Work out the finished part from the listing and answer in its coordinate system (mm). A direction names the side the tool comes from. Give positions to 0.01 mm unless a question says otherwise; leave off trailing zeros. Order: outer loops, then holes, each group sorted by start corner. A loop starts at its lowest first (then second) coordinate and runs counter-clockwise, first axis right, second up. Notation, with made-up numbers: (0.25, -0.5) - (42.25, -0.5) arc R21 ccw to (42.25, 31.5) - close; hole circle Ø5 at (-33, 42). An arc over 180 degrees is marked (long way). Write each question's results on one line, items separated by ' | '.
from build123d import *

# Parameters (mm, degrees)
F3_R = 12.7
F4_T = -2.54


with BuildPart() as f2:
    # F0 (on Front) → F2 (revolve)
    with BuildSketch(Plane.XZ):
        Polygon((0, -76.0418921709), (0, 76.0156810284), (-8.6687002331, 76.3955637813), (-8.6687002331, 59.0391717851), (-31.3122980297, 40.9342460334), (-31.3122980297, -76.0418921709), align=None)
    revolve(axis=Axis((1.9537888002, 0, -0.1578219235), (0, 0, -1)))

    # F3
    f3_edges = [f2.edges().sort_by_distance(p)[0] for p in [
        (35.219876, 0, 40.934246),
        (12.576278, 0, 59.039172),
    ]]
    fillet(f3_edges, radius=F3_R)

    # F4
    f4_openings = [f2.faces().sort_by_distance(p)[0] for p in [
        (8.241928, 0, 76.205622),
    ]]
    offset(amount=F4_T, openings=f4_openings)


solid = f2.part
1. A cutting plane is placed at B-B, the plane z = 31. Write down the section's boundary in (x, y), then the cut area to 3 significant figures.
Answer list:
outline: circle Ø66.53 at (1.95, 0); circle Ø8.99 at (1.95, 0); hole circle Ø61.45 at (1.95, 0); hole circle Ø3.91 at (1.95, 0) | area: 562 mm^2
2. Given P1, Ø3, axis at x = -6, z = -29, coming from the -Y side; P2, Ø4, axis at y = 22, z = 18, coming from the +X side; P3, Ø1, axis at x = -20.5, z = 21.5, coming from the +Y side, each flat-ended and moving along its own axis, determine where each tip first touches the part or whether it passes through.
Answer list:
P1: y = -32.63 | P2: x = 28.54 | P3: y = 24.99
3. Determine the mould class of faces 4 (the face through (-29.776, 9.992, -21.383)), 5 (the face through (2, -7, -76.042)), 6 (the face through (2, -6, -73.502)) for opening direction X: +X half, -X half, draft (parallel to the pull), parting line (faces both ways), or undercut.
Answer list:
face 4: parting line | face 5: draft | face 6: undercut
4. A cutting plane is placed at A-A, the plane z = 67. Write down the section's boundary in (x, y).
Answer list:
outline: circle Ø21.24 at (1.95, 0); circle Ø8.99 at (1.95, 0); hole circle Ø16.16 at (1.95, 0); hole circle Ø3.91 at (1.95, 0)
5. A tool of negligible diameter and unlimited length cuts with its end or side. For faces 1 (the face through (5.3, 3, 2.4)), 2 (the face through (0.15, -0.75, 1.05)), 3 (the face through (13.56, -8.899, 52.587)), from which of +Z, -Z, +X, -X, +Y, -Y can it reach the whole face along a straight path? Write none if from no direction.
Answer list:
face 1: +Z | face 2: +Z, -Z | face 3: none
6. Straight lines are drawn through the part: line 1 (Y direction, x = -1, z = -10.5); line 2 (X direction, y = -23.5, z = -13); line 3 (Z direction, x = 14, y = -7). For each, find the intervals that lie inside material, in ascending order. Write a range as [from, to].
Answer list:
line 1: [-33.13, -30.58], [-3.39, 3.39], [30.58, 33.13] | line 2: [-21.59, -17.84], [21.75, 25.5] | line 3: [-76.04, -73.5], [53.14, 56.59]
